Source: CAD feature listing. Evaluate the final solid. Frame: model axes, mm. A direction names the side the tool comes from. Give positions to 0.01 mm unless a question says otherwise; leave off trailing zeros. Order: outer loops, then holes, each group sorted by start corner. A loop starts at its lowest first (then second) coordinate and runs counter-clockwise, first axis right, second up. Notation, with made-up numbers: (82, -2) -> (117, -2) arc R13 ccw to (117, 14) -> close; hole circle Ø2 at (51.5, -3.75). An arc over 180 degrees is marked (long way). Answer in a Markdown table with one row per item.
```python
from build123d import *

# Parameters (mm, degrees)
BRKT_4_5_BOSS_EXTRUDE1_START = -60
BRKT_4_5_BOSS_EXTRUDE1_DEPTH = 120
BOSS_EXTRUDE1_DEPTH          = 8


# Read off the part's stored shape, not the designer's step: <BRKT_4_5>-<Boss-Extrude1>
with BuildPart() as part:
    # <BRKT_4_5>-<Boss-Extrude1> outline → <BRKT_4_5>-<Boss-Extrude1> (new body)
    with BuildSketch(Plane.XY.offset(BRKT_4_5_BOSS_EXTRUDE1_START)):
        Polygon((0, 0), (0, -50), (8, -50), (8, -1.773557301), (28.381375383, 41.934443258), (21.130913087, 45.315389352), align=None)
    extrude(amount=BRKT_4_5_BOSS_EXTRUDE1_DEPTH)

    # Sketch1 → Boss-Extrude1 (add)
    with BuildSketch(Plane(origin=(0, 0, -60), x_dir=(-1, 0, 0), z_dir=(0, 0, -1))):
        Polygon((-28.381375383, 41.934443258), (-21.130913087, 45.315389352), (40, 45.315389352), (40, -50), (0, -50), (-8, -50), (-8, -1.773557301), align=None)
    extrude(amount=BOSS_EXTRUDE1_DEPTH)


solid = part.part
```
(1) Section query D-D (x = 24.5). Return the cut outline in (y, z), plus the area to 3 significant figures.
A:
| item | result |
|---|---|
| outline | (33.61, -68) -> (43.74, -68) -> (43.74, 60) -> (33.61, 60) -> close |
| area | 1,300 mm^2 |
(2) Section query C-C (y = -37). Return the cut outline in (x, z).
A:
| item | result |
|---|---|
| outline | (-40, -68) -> (8, -68) -> (8, 60) -> (0, 60) -> (0, -60) -> (-40, -60) -> close |
(3) Section query A-A (z = 21.5). Return the cut outline in (x, y).
A:
| item | result |
|---|---|
| outline | (0, -50) -> (8, -50) -> (8, -1.77) -> (28.38, 41.93) -> (21.13, 45.32) -> (0, 0) -> close |
(4) Access query for faces 1 (the flat face through (8, -26, -3)), 2 (the flat face through (10.71, 22.97, -0.84)), 3 (the flat face through (0, -25, -1)). Directions: +Z, -Z, +X, -X, +Y, -Y. A direction counts if a zero-diameter tool reaches every point of the face in a straight line with its end or side. Return the directions, or none.
A:
| item | result |
|---|---|
| face 1 | +Z, -Z, +X, -Y |
| face 2 | +Z, -X, +Y |
| face 3 | +Z, -X, +Y, -Y |
(5) Section query B-B (x = -32.5). Return the cut outline in (y, z), plus the area to 3 significant figures.
A:
| item | result |
|---|---|
| outline | (-50, -68) -> (45.32, -68) -> (45.32, -60) -> (-50, -60) -> close |
| area | 763 mm^2 |
(6) First-contact query: pin 1 Ø18.5 at (x, y) = (-3.5, 21) entering from +Z; pin 2 Ø8 at (x, z) = (-2, 31.5) entering from +Y; pin 3 Ø8 at (y, z) = (20, -47) entering from +X. Flat tips, straight axial feed; report the tip coordinate or a pass-through.
A:
| item | result |
|---|---|
| pin 1 | stops at z = -60 |
| pin 2 | stops at y = 4.29 |
| pin 3 | stops at x = 20.02 |
(7) Ray query, probe 1 along Z at (x, y) = (-3, -32); probe 2 along X at (y, z) = (-17, 5); probe 3 along Y at (x, z) = (7, -11). Return the intervals inside material, ascending.
A:
| item | result |
|---|---|
| probe 1 | z = -68 to -60 |
| probe 2 | x = 0 to 8 |
| probe 3 | y = -50 to 15.01 |
